```python
from build123d import *

# Parameters (mm, degrees)
BOSS_EXTRUDE1_DEPTH = 300
SKETCH2_R           = 47.5
CUT_EXTRUDE1_DEPTH  = 100
SKETCH3_R           = 10
CUT_EXTRUDE3_REACH  = 364.052


with BuildPart() as part:
    # Sketch1 → Boss-Extrude1 (new body)
    with BuildSketch(Plane.XY):
        Polygon((94.938651754, 94.603319173), (60.438651754, 94.603319173), (60.438651754, 119.103319173), (-69.061348246, 119.103319173), (-69.061348246, -92.896680827), (60.438651754, -92.896680827), (60.438651754, -68.396680827), (94.938651754, -68.396680827), align=None)
    extrude(amount=BOSS_EXTRUDE1_DEPTH)

    # Sketch2 → Cut-Extrude1 (cut)
    with BuildSketch(Plane(origin=(94.938651754, 0, 0), x_dir=(0, 0, -1), z_dir=(1, 0, 0))):
        with Locations((-150, 13.103319173)):
            Circle(SKETCH2_R)
    extrude(amount=-CUT_EXTRUDE1_DEPTH, mode=Mode.SUBTRACT)

    # Cut-Sweep1: sweep along a path in Sketch5
    with BuildLine(Plane(origin=(25, 0, 0), x_dir=(0, 0, -1), z_dir=(1, 0, 0))) as cut_sweep1_path:
        ThreePointArc((-120, -23.723980484), (-150, 60.603319173), (-180, -23.723980484))
    # Sketch3 → Cut-Sweep1 (sweep, cut)
    with BuildSketch(Plane.XY.offset(150)):
        with Locations((24.938651754, 60.373071265)):
            Circle(SKETCH3_R)
    sweep(path=cut_sweep1_path.line, mode=Mode.SUBTRACT)

    # Cut-Extrude3: up to this face of the body (flat: up to its plane)
    cut_extrude3_end = Plane(part.part.faces().sort_by_distance((-5.061348246, 13.103319173, 150))[0])
    # Sketch7 → Cut-Extrude3 (cut, up to the picked face)
    with BuildSketch(Plane(origin=(94.938651754, 0, 0), x_dir=(0, 0, -1), z_dir=(1, 0, 0)), mode=Mode.PRIVATE) as cut_extrude3_sk1:
        with BuildLine():
            Line((-180, -23.723980484), (-186.170369742, -31.298582333))
            ThreePointArc((-186.170369742, -31.298582333), (-150, -44.166432919), (-113.829630258, -31.298582333))
            Line((-113.829630258, -31.298582333), (-120, -23.723980484))
            ThreePointArc((-120, -23.723980484), (-150, -34.396680827), (-180, -23.723980484))
        make_face()
    cut_extrude3_tool1 = split(extrude(cut_extrude3_sk1.sketch, amount=-CUT_EXTRUDE3_REACH, mode=Mode.PRIVATE), bisect_by=cut_extrude3_end, keep=Keep.BOTH, mode=Mode.PRIVATE)
    add(cut_extrude3_tool1.solids().sort_by(Axis((94.938652, -35.436268, 150), (-1, 0, 0)))[0], mode=Mode.SUBTRACT)


solid = part.part
```
Model file for the job. Use its own axes, mm. A direction names the side the tool comes from. Coordinates: 2 decimals unless noted, no trailing zeros. Write each loop counter-clockwise with the first axis right and the second up, starting at its lowest first coordinate (ties: lowest second). Pieces come first, ordered by that corner, then holes. Notation, with made-up numbers: (18, 78) - (59, 78) arc R15 ccw to (59, 92) - close; hole circle Ø1 at (-30.75, -12). An arc over 180 degrees is marked (long way). One line per item, written item: value. Start each with the question number.
1. Flat gauge pins, fed straight in: pin 1 (10 mm diameter, centred on x = -47, y = 47.5, fed in from -Z); pin 2 (19.5 mm diameter, centred on y = 110.5, z = 128, fed in from +X). Where does each tip first touch, or does it go through?
2. Tool access for faces 1 (the flat face through (94.939, 48, 115)), 2 (the flat face through (-3, 119.103, 148)), 3 (the flat face through (78, 94.603, 148)), 4 (the flat face through (77, -68.397, 148)), 5 (the flat face through (-5.061, 9, 151)): list every direction of +Z, -Z, +X, -X, +Y, -Y with a clear straight run to the whole face (end or side of a thin tool).
3. Mould opens along X. For faces 6 (the flat face through (60.439, 107, 148)), 7 (the flat face through (12, 15, 0)), 8 (the flat face through (-69.061, 15, 148)) say: released by +X, released by -X, zero draft, split by the parting line, or undercut.
4. Slice it at C-C (z = 242.5). Write the cut outline in (x, y).
5. Slice it at B-B (z = 150). Write the cut outline in (x, y), plus the area to 3 significant figures.
6. Probe line 1 (Y direction, x = 6, z = 182); line 2 (Y direction, x = 81.5, z = 150); line 3 (X direction, y = 25.5, z = 186). List the from-to ranges inside material, lowest first. Write a range as from..to.
7. Slice it at A-A (x = 51). Write the cut outline in (y, z).
Answers below:
1. pin 1: stops at z = 0
1. pin 2: stops at x = 60.44
2. face 1: +Z, -Z, +X, +Y, -Y
2. face 2: +Z, -Z, +X, -X, +Y
2. face 3: +Z, -Z, +X, +Y
2. face 4: +Z, -Z, +X, -Y
2. face 5: +X
3. face 6: released by +X
3. face 7: zero draft
3. face 8: released by -X
4. outline: (-69.06, -92.9) - (60.44, -92.9) - (60.44, -68.4) - (94.94, -68.4) - (94.94, 94.6) - (60.44, 94.6) - (60.44, 119.1) - (-69.06, 119.1) - close
5. outline: (-69.06, -92.9) - (60.44, -92.9) - (60.44, -68.4) - (94.94, -68.4) - (94.94, -44.17) - (-5.06, -44.17) - (-5.06, 60.6) - (14.94, 60.6) arc R10 cw to (34.94, 60.6) - (94.94, 60.6) - (94.94, 94.6) - (60.44, 94.6) - (60.44, 119.1) - (-69.06, 119.1) - close
5. area: 22,400 mm^2
6. line 1: y = -92.9..-34.39, -26.18..-22, 48.21..119.1
6. line 2: y = -68.4..-44.17, 60.6..94.6
6. line 3: x = -69.06..-5.06
7. outline: (-92.9, 0) - (119.1, 0) - (119.1, 300) - (-92.9, 300) - close; hole (-31.3, 113.83) - (-23.72, 120) arc R47.5 ccw (long way) to (-23.72, 180) - (-31.3, 186.17) arc R57.27 ccw to start
